```python
from build123d import *

# Parameters (mm, degrees)
SKETCH1_W           = 3
SKETCH1_H           = 24
BOSS_EXTRUDE1_DEPTH = 23
SKETCH2_W           = 6
SKETCH2_H           = 24
BOSS_EXTRUDE2_DEPTH = 2
SKETCH4_W           = 3
SKETCH4_H           = 24
BOSS_EXTRUDE3_DEPTH = 2
SKETCH5_W           = 24
SKETCH5_H           = 27
CUT_EXTRUDE1_DEPTH  = 0.5
SKETCH6_W           = 2.5
SKETCH6_H           = 24
BOSS_EXTRUDE4_DEPTH = 1


with BuildPart() as part:
    # Sketch1 → Boss-Extrude1 (new body)
    with BuildSketch(Plane(origin=(0, 0, 0), x_dir=(1, 0, 0), z_dir=(0, 1, 0))):
        with Locations((1.5, 12)):
            Rectangle(SKETCH1_W, SKETCH1_H)
    extrude(amount=BOSS_EXTRUDE1_DEPTH)

    # Sketch2 → Boss-Extrude2 (add)
    with BuildSketch(Plane(origin=(0, 23, 0), x_dir=(1, 0, 0), z_dir=(0, 1, 0))):
        with Locations((0, 12)):
            Rectangle(SKETCH2_W, SKETCH2_H)
    extrude(amount=BOSS_EXTRUDE2_DEPTH)

    # Sketch4 → Boss-Extrude3 (add)
    with BuildSketch(Plane.XZ):
        with Locations((1.5, -12)):
            Rectangle(SKETCH4_W, SKETCH4_H)
    extrude(amount=BOSS_EXTRUDE3_DEPTH)

    # Sketch5 → Cut-Extrude1 (cut)
    with BuildSketch(Plane(origin=(3, 0, 0), x_dir=(0, 0, -1), z_dir=(1, 0, 0))):
        with Locations((12, 11.5)):
            Rectangle(SKETCH5_W, SKETCH5_H)
    extrude(amount=-CUT_EXTRUDE1_DEPTH, mode=Mode.SUBTRACT)

    # Sketch6 → Boss-Extrude4 (add)
    with BuildSketch(Plane.XZ.offset(2)):
        with Locations((1.25, -12)):
            Rectangle(SKETCH6_W, SKETCH6_H)
    extrude(amount=BOSS_EXTRUDE4_DEPTH)


solid = part.part
```
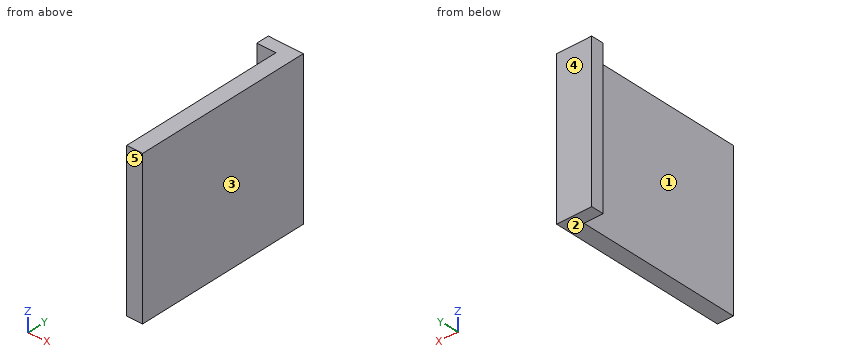
Design review of the part built by this model. Coordinates are the model's own, in mm. Face numbers are marked on the shaded views. A direction names the side the tool comes from. Coordinates: 2 decimals unless noted, no trailing zeros. Loops run counter-clockwise (first coordinate to the right, second up) from the corner with the lowest first, then second, coordinate; pieces in that order, holes last.
Q1. We need section B-B on x = -0.35. State the section outline as (y, z) points, and give its area (3 significant figures).
Reported:
outline: (23, -24) - (25, -24) - (25, 0) - (23, 0) - close
area: 48.0 mm2
Q2. The part is to be moulded in two halves that separate along Y. For the marked faces 3, 4 and 5, say which applies: +Y half, -Y half, draft (parallel to the pull), parting line (faces both ways), or undercut.
Reported:
face 3: draft
face 4: +Y half
face 5: -Y half
Q3. For pin 1 (7 mm diameter, centred on y = 10, z = -16, fed in from -X); pin 2 (2 mm diameter, centred on x = -2, y = 8, fed in from -Z); pin 3 (1.5 mm diameter, centred on x = -1, z = -16, fed in from -Y), all flat-tipped, find the tip position at first contact; note any pin that passes through.
Reported:
pin 1: stops at x = 0
pin 2: passes through
pin 3: stops at y = 23
Q4. We need section A-A on z = -7. State the section outline as (x, y) points, and give its area (3 significant figures).
Reported:
outline: (-3, 23) - (0, 23) - (0, -3) - (2.5, -3) - (2.5, 25) - (-3, 25) - close
area: 76.0 mm2
Q5. To check wall thickness, follow line 1 (X direction, y = -0.5, z = -20); line 2 (Y direction, x = -2.25, z = -12). State the ranges of each line that lie inside material, in increasing order.
Reported:
line 1: x = 0 to 2.5
line 2: y = 23 to 25
Q6. We need section C-C on y = -1. State the section outline as (x, z) points.
Reported:
outline: (0, -24) - (2.5, -24) - (2.5, 0) - (0, 0) - close
Q7. Tool access review of the marked faces 1 and 2: name each direction out of +Z, -Z, +X, -X, +Y, -Y from which nothing blocks a thin tool from reaching the whole face with its end or side.
Reported:
face 1: +Z, -Z, -X, -Y
face 2: -Z, +X, -X, +Y, -Y
